Verification items for the finished model (mm, model axes). A direction names the side the tool comes from. Coordinates: 2 decimals unless noted, no trailing zeros. Order: outer loops, then holes, each group sorted by start corner. A loop starts at its lowest first (then second) coordinate and runs counter-clockwise, first axis right, second up. Notation, with made-up numbers: (-9, -28) - (11, -28) arc R34 ccw to (11, 7) - close; hole circle Ø2 at (66, 53.25). An arc over 180 degrees is marked (long way). Answer as CSV lines item,"result". Start each with the question number.
1. Section check D-D (x = -12). Record the cut outline in (y, z), and give its area (3 significant figures).
2. Set-up check for faces 4 (the flat face through (-3, -18.97, -9)), 5 (the flat face through (5.25, -16.63, -13.04)), 6 (the flat face through (-13.1, -16.63, 5.3)), 7 (the flat face through (5.2, -16.63, 13.1)), 8 (the flat face through (-6, -16.63, -13)): record each of +Z, -Z, +X, -X, +Y, -Y from which the full face is reachable in a straight line by a thin tool's end or side.
3. Section check B-B (z = -2). Record the cut outline in (x, y).
4. Material ranges on L1, parallel to X at y = -17.3, z = 0; L2, parallel to Z at x = 0, y = -26.25; L3, parallel to Z at x = 0, y = -21, recorded low to high. Write a range as [from, to].
5. Mould release check, pull along Z, two halves, no side actions. Record for faces 1 (the cylindrical face through (5, -25.84, 7.84)), 2 (the flat face through (1, -18.5, -7)), 3 (the flat face through (-13.1, -16.63, -5.2)): pulls with the +Z half, pulls with the -Z half, needs draft (parallel to the pull), parting line crosses it, or undercut.
6. Section check C-C (y = -26.5). Record the cut outline in (x, z).
7. Section check A-A (x = -4.5). Record the cut outline in (y, z).
8. Go/stop test with flat-tipped pins: pin 1 (3.5 mm diameter, centred on x = 6, z = -11.5, fed in from +Y); pin 2 (4.5 mm diameter, centred on x = 6.5, z = -11, fed in from -Y); pin 3 (3 mm diameter, centred on y = -10.5, z = -4, fed in from +X); pin 4 (12 mm diameter, centred on x = 9.5, y = -7.5, fed in from +Z). Record where each tip stops, or that it passes through.
Autodesk Inventor part; units mm, degrees
ref_plane "Plano de trabajo2" through (0, -18.5, 0) normal (0, 1, 0) x (1, 0, 0)
ref_plane "YZ Plane" through (0, 0, 0) normal (1, 0, 0) x (0, 1, 0)
ref_plane "XZ Plane" through (0, 0, 0) normal (0, 1, 0) x (-1, 0, 0)
sketch "Boceto1" plane through (0, 0, 0) normal (0, 1, 0) x (-1, 0, 0)
  circle A0 centre (0, 0) radius 10.7
  circle A1 centre (0, 0) radius 13.88
  dimension "d0" = 21.4
  dimension "d1" = 27.76
extrude "Extrusión1" add sketch "Boceto1" against normal blind 22.6
sketch "Boceto2" plane through (0, -22.6, 0) normal (0, -1, 0) x (1, 0, 0)
  circle A0 centre (0, 0) radius 13.88
  line L0 (0, -13.88) -> (-5.75, -13.88)
  line L1 (0, -13.88) -> (5.75, -13.88)
  line L2 (13.88, 0) -> (13.88, -5.75)
  line L3 (13.88, 0) -> (13.88, 5.75)
  line L4 (0, 13.88) -> (5.75, 13.88)
  line L5 (0, 13.88) -> (-5.75, 13.88)
  line L6 (-13.88, 0) -> (-13.88, -5.75)
  line L7 (-13.88, 0) -> (-13.88, 5.75)
  line L8 (-13.88, 5.75) -> (-5.75, 13.88)
  line L9 (5.75, 13.88) -> (13.88, 5.75)
  line L10 (13.88, -5.75) -> (5.75, -13.88)
  line L11 (-5.75, -13.88) -> (-13.88, -5.75)
  dimension "d5" = 5.75
  dimension "d6" = 5.75
  dimension "d7" = 5.75
  dimension "d8" = 5.75
  dimension "d9" = 5.75
  dimension "d10" = 5.75
  dimension "d11" = 5.75
  dimension "d12" = 5.75
extrude "Extrusión2" add sketch "Boceto2" against normal blind 5.97
ref_plane "Plano de trabajo2" through (0, -18.5, 0) normal (0, 1, 0) x (1, 0, 0)
sketch "Boceto4" plane through (0, -18.5, 0) normal (0, 1, 0) x (1, 0, 0)
  circle A0 centre (0, 0) radius 6.8
  dimension "d18" = 13.6
extrude "Extrusión4" add sketch "Boceto4" against normal blind 18.97
sketch "Boceto5" plane through (0, 0, 0) normal (0, 1, 0) x (1, 0, 0)
  circle A0 centre (0, 0) radius 10.7
extrude "Extrusión5" cut sketch "Boceto5" against normal blind 18.97
sketch "Boceto6" plane through (0, -37.47, 0) normal (0, -1, 0) x (1, 0, 0)
  circle A0 centre (0, 0) radius 6.7
  circle A1 centre (0, 0) radius 9.3
  dimension "d25" = 13.4
  dimension "d26" = 18.6
extrude "Extrusión6" add sketch "Boceto6" against normal blind 18.97
sketch "Boceto7" plane through (0, -37.47, 0) normal (0, -1, 0) x (1, 0, 0)
  circle A0 centre (0, 0) radius 6.8
  dimension "d29" = 13.6
extrude "Extrusión7" cut sketch "Boceto7" against normal blind 18.97
thread "Rosca2"
sketch "Boceto9" plane through (0, -37.47, 0) normal (0, -1, 0) x (1, 0, 0)
  circle A0 centre (0, 0) radius 9.3
extrude "Extrusión8" cut sketch "Boceto9" against normal blind 8.47
properties part number "ACOPLE2"
Evaluation:
1,outline,"(-22.6, -7.63) - (-16.63, -7.63) - (-16.63, -6.98) - (0, -6.98) - (0, 6.98) - (-16.63, 6.98) - (-16.63, 7.63) - (-22.6, 7.63) - close"
1,area,"323 mm²"
2,face 4,"+Y"
2,face 5,"-Z, +X, +Y"
2,face 6,"+Z, -X, +Y"
2,face 7,"+Z, +X, +Y"
2,face 8,"-Z, -X, +Y"
3,outline,"(-13.88, -22.6) - (-9.08, -22.6) - (-9.08, -29) - (-6.5, -29) - (-6.5, -18.5) - (-9.08, -18.5) - (-9.08, -18.97) - (-10.51, -18.97) - (-10.51, 0) - (-13.74, 0) - (-13.74, -16.63) - (-13.88, -16.63) - close; (6.5, -29) - (9.08, -29) - (9.08, -22.6) - (13.88, -22.6) - (13.88, -16.63) - (13.74, -16.63) - (13.74, 0) - (10.51, 0) - (10.51, -18.97) - (9.08, -18.97) - (9.08, -18.5) - (6.5, -18.5) - close"
4,L1,"x = [-13.88, -10.7], [10.7, 13.88]"
4,L2,"z = [-9.3, -6.8], [6.8, 9.3]"
4,L3,"z = [-13.88, -6.8], [6.8, 13.88]"
5,face 1,"parting line crosses it"
5,face 2,"undercut"
5,face 3,"needs draft"
6,outline,"circle Ø18.6 at (0, 0); hole circle Ø13.6 at (0, 0)"
7,outline,"(-29, -8.14) - (-22.6, -8.14) - (-22.6, -13.88) - (-16.63, -13.88) - (-16.63, -13.13) - (0, -13.13) - (0, -9.71) - (-18.97, -9.71) - (-18.97, -8.14) - (-18.5, -8.14) - (-18.5, -5.1) - (-29, -5.1) - close; (-29, 5.1) - (-18.5, 5.1) - (-18.5, 8.14) - (-18.97, 8.14) - (-18.97, 9.71) - (0, 9.71) - (0, 13.13) - (-16.63, 13.13) - (-16.63, 13.88) - (-22.6, 13.88) - (-22.6, 8.14) - (-29, 8.14) - close"
8,pin 1,"stops at y = 0"
8,pin 2,"stops at y = -22.6"
8,pin 3,"stops at x = 13.65"
8,pin 4,"stops at z = 13.43"
